Verification items for this drawing (mm, ordinates from the low corner). A direction names the side the tool comes from. Round coordinates to 2 decimals unless told otherwise and drop trailing zeros. Loops run counter-clockwise (first coordinate to the right, second up) from the corner with the lowest first, then second, coordinate; pieces in that order, holes last. Notation, with made-up numbers: (-36.75, 19.5) - (16.25, 19.5) arc R19 cw to (16.25, 54.5) - close; hole circle Ø3 at (7.5, 19.25). An arc over 180 degrees is marked (long way). Answer in a Markdown table with one row per item. Add a question column.
(1) Mould release check, pull along X, two halves, no side actions. Record for the marked faces 4, 5 and 6: +X half, -X half, draft (parallel to the pull), parting line (faces both ways), or undercut.
(2) Gauge pin test, flat ends, axial feed: pin 1 (3 mm diameter, centred on x = 1, y = 37.5, fed in from -Z); pin 2 (6 mm diameter, centred on y = 51, z = 27, fed in from -X); pin 3 (1.5 mm diameter, centred on x = 24, y = 73.5, fed in from +Z) (1 decimal); pin 4 (12 mm diameter, centred on x = 6.5, z = 62, fed in from +Y). Record the tip position at first contact, or that the pin passes through.
(3) Thickness scan on line 1 along X through (y, z) = (4, 55); line 2 along Z through (x, y) = (5, 12.5); line 3 along X through (y, z) = (61, 20). Record the ranges inside material, lowest first.
(4) Cross-section at D-D on x = 41. Enter the section's corners in (y, z).
(5) Cross-section at A-A on z = 5. Enter the section's corners in (x, y) (1 decimal).
(6) Access from +Z, -Z, +X, -X, +Y, -Y to the whole of each face (thin tool, end or side, straight path). Record for the marked faces 1, 2 and 3.
(7) Cross-section at C-C on z = 40.5. Enter the section's corners in (x, y).
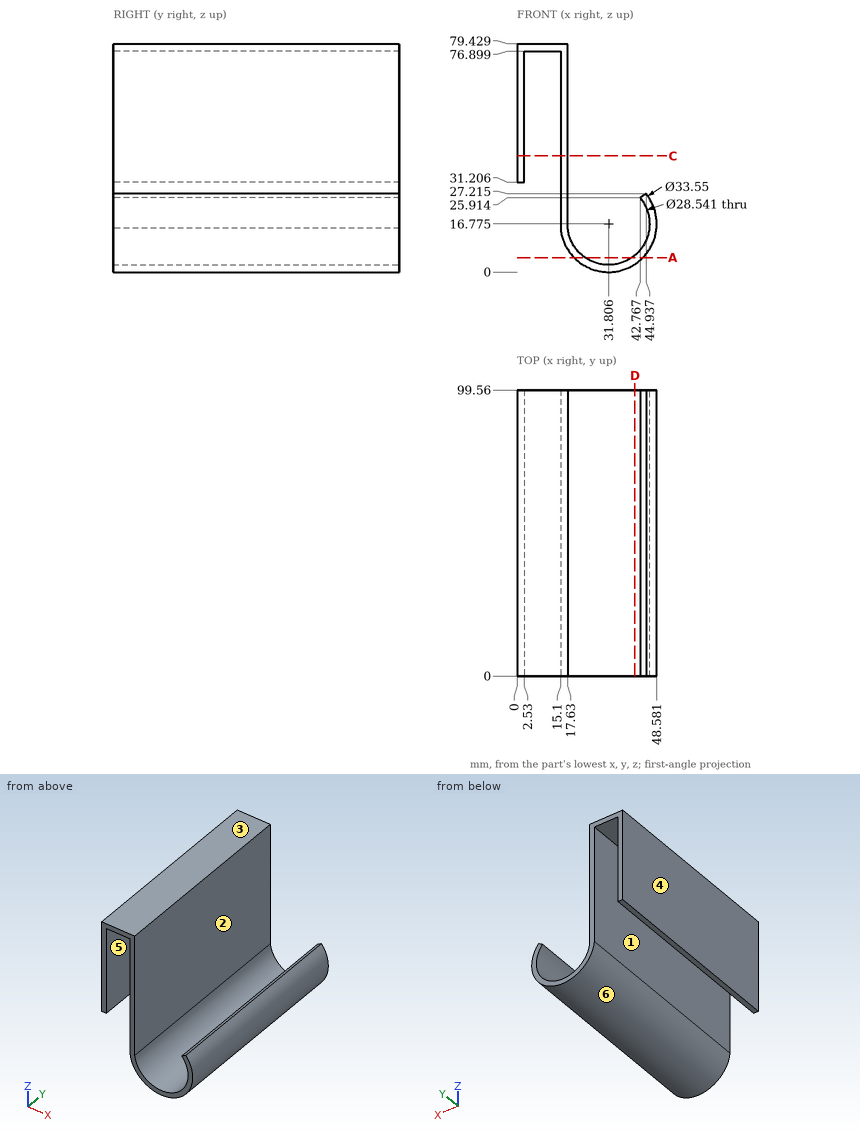
Answers:
| question | item | result |
|---|---|---|
| 1 | face 4 | -X half |
| 1 | face 5 | undercut |
| 1 | face 6 | parting line |
| 2 | pin 1 | stops at z = 31.21 |
| 2 | pin 2 | stops at x = 15.1 |
| 2 | pin 3 | stops at z = 5.4 |
| 2 | pin 4 | stops at y = 99.56 |
| 3 | line 1 | x = 0 to 2.53, 15.1 to 17.63 |
| 3 | line 2 | z = 76.9 to 79.43 |
| 3 | line 3 | x = 15.1 to 17.63, 45.71 to 48.27 |
| 4 | outline | (0, 2.74) - (99.56, 2.74) - (99.56, 5.86) - (0, 5.86) - close |
| 5 | outline | (19.9, 0) - (23.7, 0) - (23.7, 99.6) - (19.9, 99.6) - close; (39.9, 0) - (43.8, 0) - (43.8, 99.6) - (39.9, 99.6) - close |
| 6 | face 1 | -Z, +Y, -Y |
| 6 | face 2 | +Z, +Y, -Y |
| 6 | face 3 | +Z, +X, -X, +Y, -Y |
| 7 | outline | (0, 0) - (2.53, 0) - (2.53, 99.56) - (0, 99.56) - close; (15.1, 0) - (17.63, 0) - (17.63, 99.56) - (15.1, 99.56) - close |
